For this review, take the finished solid that the model builds, in its own axes (mm). A direction names the side the tool comes from. Give positions to 0.01 mm unless a question says otherwise; leave off trailing zeros. Loops run counter-clockwise (first coordinate to the right, second up) from the corner with the lowest first, then second, coordinate; pieces in that order, holes last.
```python
from build123d import *

# Parameters (mm, degrees)
F0_W     = 113.03
F0_H     = 25.4
F1_DEPTH = 6.35
F2_R     = 3.81
F3_DEPTH = 6.351
F4_W     = 12.7
F4_H     = 25.4
F5_DEPTH = 12.7
F6_R     = 1.8288
F7_DEPTH = 254


with BuildPart() as f1:
    # F0 (on Top) → F1 (new body)
    with BuildSketch(Plane.XY):
        Rectangle(F0_W, F0_H)
    extrude(amount=F1_DEPTH)

    # F2 (on face) → F3 (cut, through all)
    with BuildSketch(Plane.XY.offset(6.35)):
        Circle(F2_R)
    extrude(amount=-F3_DEPTH, mode=Mode.SUBTRACT)

    # F4 (on face) → F5 (join)
    with BuildSketch(Plane(origin=(0, 0, 0), x_dir=(1, 0, 0), z_dir=(0, 0, -1))):
        with Locations((-50.165, 0)):
            Rectangle(F4_W, F4_H)
        with Locations((50.165, 0)):
            Rectangle(F4_W, F4_H)
    extrude(amount=F5_DEPTH)

    # F6 (on face) → F7 (cut)
    with BuildSketch(Plane(origin=(-56.515, 0, 0), x_dir=(0, -1, 0), z_dir=(-1, 0, 0))):
        with Locations((-6.35, -6.35)):
            Circle(F6_R)
        with Locations((6.35, -6.35)):
            Circle(F6_R)
    extrude(amount=-F7_DEPTH, mode=Mode.SUBTRACT)


solid = f1.part
```
Item 1: The part is to be moulded in two halves that separate along X. For faces 3 (the flat face through (-43.815, 0, -6)), 4 (the flat face through (-56.515, 0, -3)), 5 (the cylindrical face through (-0.83, -3.72, 3.22)), 6 (the flat face through (50, 0, -12.7)), say which applies: released by +X, released by -X, zero draft, split by the parting line, or undercut.
Answer:
face 3: undercut
face 4: released by -X
face 5: undercut
face 6: zero draft
Item 2: Tool access review of faces 1 (the flat face through (43.815, 0, -6)), 2 (the cylindrical face through (-50.254, -5.954, -8.135)): name each direction out of +Z, -Z, +X, -X, +Y, -Y from which nothing blocks a thin tool from reaching the whole face with its end or side.
Answer:
face 1: -Z, +Y, -Y
face 2: +X, -X
Item 3: For L1, parallel to X at y = 9.5, z = -8.5 (3 decimals); L2, parallel to Y at x = -46, z = -8; L3, parallel to Z at x = 36, y = -2.75, list the stretches that pass through material, from the lowest coordinate up.
Answer:
L1: x = -56.515 to -43.815, 43.815 to 56.515
L2: y = -12.7 to -7.14, -5.56 to 5.56, 7.14 to 12.7
L3: z = 0 to 6.35
Item 4: Take a section at C-C on x = 0. Give the boundary of the cut face in (y, z), and give its area (3 significant figures).
Answer:
outline: (-12.7, 0) - (-3.81, 0) - (-3.81, 6.35) - (-12.7, 6.35) - close; (3.81, 0) - (12.7, 0) - (12.7, 6.35) - (3.81, 6.35) - close
area: 113 mm2
Item 5: Take a section at D-D on z = -1.75. Give the boundary of the cut face in (x, y) (3 decimals), and give its area (3 significant figures).
Answer:
outline: (-56.515, -12.7) - (-43.815, -12.7) - (-43.815, 12.7) - (-56.515, 12.7) - close; (43.815, -12.7) - (56.515, -12.7) - (56.515, 12.7) - (43.815, 12.7) - close
area: 645 mm2
Item 6: Clearance check with flat-ended pins moving along their axes: pin 1 Ø2 at (y, z) = (-6.35, -6.35) entering from +X; pin 2 Ø4 at (x, y) = (-33.5, -2.5) entering from -Z. State where each tip first meets the part, or that it passes through.
Answer:
pin 1: passes through
pin 2: stops at z = 0
Item 7: Take a section at B-B on y = 6.35. Give the boundary of the cut face in (x, z) (3 decimals).
Answer:
outline: (-56.515, -12.7) - (-43.815, -12.7) - (-43.815, -8.179) - (-56.515, -8.179) - close; (-56.515, -4.521) - (-43.815, -4.521) - (-43.815, 0) - (43.815, 0) - (43.815, -4.521) - (56.515, -4.521) - (56.515, 6.35) - (-56.515, 6.35) - close; (43.815, -12.7) - (56.515, -12.7) - (56.515, -8.179) - (43.815, -8.179) - close
Item 8: Take a section at A-A on z = -6.35. Give the boundary of the cut face in (x, y) (3 decimals), and give its area (3 significant figures).
Answer:
outline: (-56.515, -12.7) - (-43.815, -12.7) - (-43.815, -8.179) - (-56.515, -8.179) - close; (-56.515, -4.521) - (-43.815, -4.521) - (-43.815, 4.521) - (-56.515, 4.521) - close; (-56.515, 8.179) - (-43.815, 8.179) - (-43.815, 12.7) - (-56.515, 12.7) - close; (43.815, -12.7) - (56.515, -12.7) - (56.515, -8.179) - (43.815, -8.179) - close; (43.815, -4.521) - (56.515, -4.521) - (56.515, 4.521) - (43.815, 4.521) - close; (43.815, 8.179) - (56.515, 8.179) - (56.515, 12.7) - (43.815, 12.7) - close
area: 459 mm2
